```python
from build123d import *

# Parameters (mm, degrees)
BOSS_EXTRUDE2_DEPTH = 3
BOSS_EXTRUDE3_DEPTH = 3
CHAMFER1_SIZE       = 1.5
BOSS_EXTRUDE4_DEPTH = 3
CUT_EXTRUDE1_DEPTH  = 1
CHAMFER2_SIZE       = 1


with BuildPart() as part:
    # Sketch1 → Boss-Extrude2 (new body)
    with BuildSketch(Plane(origin=(0, 0, 0), x_dir=(1, 0, 0), z_dir=(0, 1, 0))):
        Polygon((-3.617228643129947, -6.5e-16), (-1.8086143215649655, -3.132611896247254), (1.8086143215649881, -3.132611896247241), (3.6172286431299465, 2.591e-14), (1.8086143215649435, 3.132611896247266), (-1.8086143215650103, 3.1326118962472274), align=None)
        Polygon((1.9999999999999936, 0.8284271247461886), (0.8284271247461865, 1.999999999999994), (-0.8284271247461888, 1.9999999999999927), (-1.9999999999999936, 0.8284271247461867), (-1.9999999999999922, -0.8284271247461881), (-0.8284271247461862, -1.9999999999999931), (0.8284271247461892, -1.9999999999999918), (1.999999999999994, -0.8284271247461859), align=None, mode=Mode.SUBTRACT)
    extrude(amount=BOSS_EXTRUDE2_DEPTH)

    # Sketch3 → Boss-Extrude3 (add)
    with BuildSketch(Plane(origin=(0, 0, 0), x_dir=(1, 0, 0), z_dir=(0, 1, 0))):
        Polygon((1.35009e-12, -6.265223792495006), (3.191385678434759, -11.792865934089827), (1.7284641960877252, -15.524235391675447), (4.912158247964482, -21.038555245281238), (3.7655427137404005, -25.31778267575289), (0.2655427137398905, -19.25560484926116), (-7.234457286261282, -6.2652237924924865), (-9.043071607825457, -3.132611896246603), (-7.234457286259898, 1.64471e-12), (-5.425842964695981, 3.1326118962470666), (-11.808614321563178, 3.132611896247083), (-14.30861432156403, 6.265223792494697), (-20.676002425317918, 6.265223792494897), (-23.80861432156554, 9.397835688742644), (-16.808614321564708, 9.397835688742767), (-1.8086143215623112, 9.397835688742738), (1.8086143215660542, 9.397835688742727), (3.6172286431313894, 6.265223792494598), (5.4258429646954855, 3.132611896248873), (8.617228643129225, 8.660254037843819), (12.58015012547734, 9.259011599181736), (15.763844177354214, 14.77333145278746), (20.043071607826096, 15.919946987011269), (16.54307160782585, 9.857769160519384), (9.04307160782462, -3.1326118962492617), (7.234457286260429, -6.265223792495135), (3.6172286431296587, -6.265223792494937), align=None)
        Polygon((-1.8086143215639572, -3.132611896247045), (-3.617228643129372, 9.8462e-13), (-1.808614321565077, 3.1326118962470595), (1.8086143215657584, 3.1326118962474574), (3.6172286431299985, 1.0129e-12), (1.8086143215649881, -3.132611896247241), align=None, mode=Mode.SUBTRACT)
    extrude(amount=BOSS_EXTRUDE3_DEPTH)

    # Chamfer1
    chamfer1_edges = [part.edges().sort_by_distance(p)[0] for p in [
        (17.903457892590154, 3, -15.346639219899364),
        (14.171997151415777, 3, -12.016171525984598),
        (10.598689384303283, 3, -8.959632818512777),
        (7.021535803912355, 3, -5.896432967046346),
        (-22.24230837344173, 3, -7.8315297406187705),
        (-17.492308373440974, 3, -6.2652237924947976),
        (-13.058614321563603, 3, -4.69891784437089),
        (-8.617228643129579, 3, -3.1326118962470746),
        (4.338850480852441, 3, 23.178168960517063),
        (3.3203112220261035, 3, 18.281395318478342),
        (2.459924937261242, 3, 13.658550662882636),
        (1.5956928392180545, 3, 9.029044863292416),
    ]]
    chamfer(chamfer1_edges, length=CHAMFER1_SIZE)

    # Sketch4 → Boss-Extrude4 (add)
    with BuildSketch(Plane(origin=(0, 0, 0), x_dir=(1, 0, 0), z_dir=(0, 1, 0))):
        Polygon((-6.798376917342761, -0.16876811390146088), (-6.798376917342759, -6.096455678591746), (-8.026041208745289, -5.587940479051664), (-9.043071607825457, -3.132611896246603), (-8.026041208745289, -0.6772833134415445), align=None)
        Polygon((3.4264760493730018, 7.289397235314943), (1.8086143215658708, 9.39783568874193), (-0.8262778053214378, 9.744725818120022), (-1.8804970320349317, 8.935794954216455), (3.2530309846839565, 5.97195117187129), align=None)
        Polygon((4.59956515937226, -6.612113921873456), (7.23445728625957, -6.2652237924954015), (8.852319014066733, -4.156785339068437), (8.678873949377703, -2.8393392756247793), (3.545345932658778, -5.803183057969877), align=None)
    extrude(amount=BOSS_EXTRUDE4_DEPTH)

    # Sketch6 → Cut-Extrude1 (cut)
    with BuildSketch(Plane(origin=(0, 3, 0), x_dir=(1, 0, 0), z_dir=(0, 1, 0))):
        Polygon((1.058614321565864, 8.098797583065272), (-0.07961424608791523, 8.248648216822222), (-0.9904237841107939, 7.549759477388622), (-1.1402744178677426, 6.411530909734845), (-0.4413856784341425, 5.500721371711964), (0.6968428892196359, 5.350870737955016), (1.6076524272425143, 6.049759477388614), (1.757503060999463, 7.187988045042393), align=None)
        Polygon((-7.543071607825456, -3.1326118962466047), (-7.103731779605277, -4.193272068026425), (-6.043071607825456, -4.632611896246601), (-4.982411436045638, -4.193272068026424), (-4.5430716078254605, -3.1326118962466007), (-4.982411436045639, -2.071951724466782), (-6.043071607825459, -1.6326118962466047), (-7.103731779605278, -2.0719517244667833), align=None)
        Polygon((6.484457286259583, -4.966185686818733), (7.183346025693192, -4.0553761487958635), (7.033495391936258, -2.9171475811420824), (6.122685853913389, -2.218258841708473), (4.984457286259606, -2.368109475465409), (4.2855685468259965, -3.2789190134882777), (4.435419180582931, -4.417147581142059), (5.346228718605801, -5.116036320575668), align=None)
    extrude(amount=-CUT_EXTRUDE1_DEPTH, mode=Mode.SUBTRACT)

    # Chamfer2
    chamfer2_edges = [part.edges().sort_by_distance(p)[0] for p in [
        (1.2077191668051772, 3, 6.265223792494805),
        (4.821983381293134, 3, -4.1785273753389465),
        (-6.029702548098242, 3, -2.0866964171569644),
    ]]
    chamfer(chamfer2_edges, length=CHAMFER2_SIZE)


solid = part.part
```
Geometry: final body of the model. Coordinates: model frame, mm. A direction names the side the tool comes from. Round coordinates to 2 decimals unless told otherwise and drop trailing zeros. Loops run counter-clockwise (first coordinate to the right, second up) from the corner with the lowest first, then second, coordinate; pieces in that order, holes last. Notation, with made-up numbers: (33, -21) -> (76, -21) arc R9 cw to (76, -15) -> close; hole circle Ø8 at (80, -17). An arc over 180 degrees is marked (long way). Use one line per item in the form item = value. Start each with the question number.
1) Access query for faces 1 (the flat face through (0, 2, -7)), 2 (the flat face through (-7.69, 1.83, 0.54)), 3 (the flat face through (1.42, 1.48, -1.41)). Directions: +Z, -Z, +X, -X, +Y, -Y. A direction counts if a zero-diameter tool reaches every point of the face in a straight line with its end or side. Return the directions, or none.
2) Section B-B on x = -18. Output: boundary loops of the cut face in (y, z), then the cut area to 3 significant figures.
3) Draft query along X for faces 4 (the flat face through (3.298, 0.74, 18.243)), 5 (the flat face through (18.06, 2.24, -14.62)), 6 (the flat face through (-0.529, 2.507, -7.904)). Return one class per face: released by +X, released by -X, zero draft, split by the parting line, or undercut.
4) Section D-D on y = 2.5. Give the number of separate pieces and of enclosed holes in the cut face, then the cut area to 3 significant figures.
5) Section A-A on z = -1.5. Output: boundary loops of the cut face in (x, y).
6) Line query: L1, parallel to X at y = 2.85, z = 3.5; L2, parallel to Z at x = -19.5, y = 1.95; L3, parallel to X at y = 0.1, z = -3. Output: solid intervals per line, ascending.
7) First-contact query: P1, Ø0.8, axis at x = 0.5, y = 1.5, coming from the -Z side; P2, Ø1.8, axis at y = 1, z = 0, coming from the -X side; P3, Ø1, axis at x = -4.5, y = 1, coming from the +Z side; P4, Ø2, axis at x = -15, z = -3.5, coming from the +Y side. Flat tips, straight axial feed; report the tip coordinate or a pass-through.
8) Section C-C on z = 17.5. Output: boundary loops of the cut face in (x, y), then the cut area to 3 significant figures.
Response:
q1.face_1 = +Y
q1.face_2 = -X, +Y
q1.face_3 = +Y, -Y
q2.outline = (0, -9.4) -> (3, -9.4) -> (3, -7.77) -> (1.5, -6.27) -> (0, -6.27) -> close
q2.area = 8.27 mm^2
q3.face_4 = released by +X
q3.face_5 = released by -X
q3.face_6 = undercut
q4.separate_pieces = 1
q4.enclosed_holes = 4
q4.area = 352 mm^2
q5.outline = (-6.37, 0) -> (-1.33, 0) -> (-1.33, 3) -> (-5.21, 3) -> (-6.37, 2) -> close; (1.33, 0) -> (11.72, 0) -> (11.72, 3) -> (6.22, 3) -> (5.71, 2.57) -> (5.21, 3) -> (1.33, 3) -> close
q6.L1 = -8.89 to -7.39, -4.7 to 4.31, 7.11 to 8.83
q6.L2 = -9.4 to -6.72
q6.L3 = -5.5 to 12.58
q7.P1 = -9.62
q7.P2 = -8.12
q7.P3 = 11.87
q7.P4 = through
q8.outline = (-0.75, 0) -> (2.87, 0) -> (2.87, 1.5) -> (1.14, 3) -> (-0.75, 3) -> close
q8.area = 9.55 mm^2
